Can you work these out from the model? Positions are in its coordinate system, mm. Round coordinates to 2 decimals unless told otherwise and drop trailing zeros. Loops run counter-clockwise (first coordinate to the right, second up) from the corner with the lowest first, then second, coordinate; pieces in that order, holes last. Notation, with made-up numbers: (15.5, 19) -> (23.5, 19) arc R22 ccw to (23.5, 53) -> close; hole circle Ø6 at (-28, 44). An arc over 180 degrees is marked (long way). Answer as a JSON object with one key per item and string values.
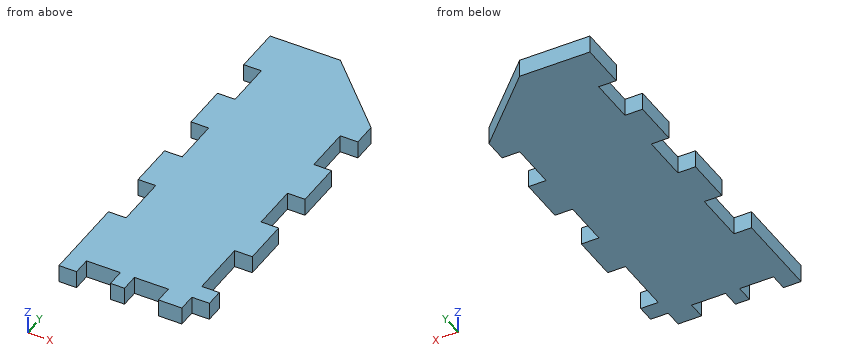
```python
from build123d import *

# Parameters (mm, degrees)
BOSS_EXTRUDE1_DEPTH = 4.7752
SKETCH3_W           = 9.1948
SKETCH3_H           = 4.7752
SKETCH3_W_2         = 4.7752
CUT_EXTRUDE4_DEPTH  = 6.35
SKETCH4_W           = 4.7752
SKETCH4_H           = 12.774972335
SKETCH4_H_2         = 12.7
SKETCH4_H_3         = 14.2748
SKETCH4_H_4         = 15.8496
SKETCH4_H_5         = 12.625027665
CUT_EXTRUDE5_DEPTH  = 6.35


with BuildPart() as part:
    # Sketch2 → Boss-Extrude1 (new body)
    with BuildSketch(Plane.XY):
        Polygon((0, 0), (0, 101.6), (19.05, 101.6), (38.1, 82.55), (38.1, 0), align=None)
    extrude(amount=BOSS_EXTRUDE1_DEPTH)

    # Sketch3 → Cut-Extrude4 (cut)
    with BuildSketch(Plane.XY.offset(4.7752)):
        with Locations((9.3726, 2.3876)):
            Rectangle(SKETCH3_W, SKETCH3_H)
        with Locations((22.3774, 2.3876)):
            Rectangle(SKETCH3_W, SKETCH3_H)
        with Locations((35.7124, 2.3876)):
            Rectangle(SKETCH3_W_2, SKETCH3_H)
    extrude(amount=-CUT_EXTRUDE4_DEPTH, mode=Mode.SUBTRACT)

    # Sketch4 → Cut-Extrude5 (cut)
    with BuildSketch(Plane.XY.offset(4.7752)):
        with Locations((2.3876, 57.187486168)):
            Rectangle(SKETCH4_W, SKETCH4_H)
        with Locations((35.7124, 44.45)):
            Rectangle(SKETCH4_W, SKETCH4_H_2)
        with Locations((2.3876, 30.9626)):
            Rectangle(SKETCH4_W, SKETCH4_H_3)
        with Locations((35.7124, 17.4752)):
            Rectangle(SKETCH4_W, SKETCH4_H_4)
        with Locations((35.7124, 69.85)):
            Rectangle(SKETCH4_W, SKETCH4_H_2)
        with Locations((2.3876, 82.587486168)):
            Rectangle(SKETCH4_W, SKETCH4_H_5)
    extrude(amount=-CUT_EXTRUDE5_DEPTH, mode=Mode.SUBTRACT)


solid = part.part
```
Q1. I want a section at A-A, the plane x = 2. Write out the boundary of the cut face in (y, z), then the cut area to 3 significant figures.
Determined:
{"outline": "(0, 0) -> (23.83, 0) -> (23.83, 4.78) -> (0, 4.78) -> close; (38.1, 0) -> (50.8, 0) -> (50.8, 4.78) -> (38.1, 4.78) -> close; (63.57, 0) -> (76.27, 0) -> (76.27, 4.78) -> (63.57, 4.78) -> close; (88.9, 0) -> (101.6, 0) -> (101.6, 4.78) -> (88.9, 4.78) -> close", "area": "296 mm²"}
Q2. I want a section at C-C, the plane x = 22.5. Write out the boundary of the cut face in (y, z), then the cut area to 3 significant figures.
Determined:
{"outline": "(4.78, 0) -> (98.15, 0) -> (98.15, 4.78) -> (4.78, 4.78) -> close", "area": "446 mm²"}
Q3. If I drill on L1, parallel to Y at x = 18, z = 3.55; L2, parallel to Y at x = 34, z = 0.2; L3, parallel to X at y = 62.5, z = 2.25, over which ranges is the centre line in solid material (lowest first)? Write a range as [from, to].
Determined:
{"L1": "[4.78, 101.6]", "L2": "[4.78, 9.55], [25.4, 38.1], [50.8, 63.5], [76.2, 86.65]", "L3": "[4.78, 38.1]"}
Q4. I'm going to push flat-ended pins straight in: pin 1 (2.5 mm diameter, centred on x = 36.5, z = 3.5, fed in from -Y); pin 2 (2.5 mm diameter, centred on y = 30, z = 1.5, fed in from -X); pin 3 (2.5 mm diameter, centred on y = 1.5, z = 3, fed in from +X); pin 4 (1.4 mm diameter, centred on x = 1.5, z = 1.5, fed in from -Y). Where does each tip first touch, or does it pass through?
Determined:
{"pin 1": "y = 4.78", "pin 2": "x = 4.78", "pin 3": "x = 33.32", "pin 4": "y = 0"}
Q5. I want a section at B-B, the plane y = 20.5. Write out the boundary of the cut face in (x, z), then the cut area to 3 significant figures.
Determined:
{"outline": "(0, 0) -> (33.32, 0) -> (33.32, 4.78) -> (0, 4.78) -> close", "area": "159 mm²"}
